from build123d import *

# Parameters (mm, degrees)
BOSS_EXTRUDE1_DEPTH      = 15
BOSS_EXTRUDE1_DEPTH_BACK = 15
SKETCH1_R                = 25
SKETCH1_R_2              = 6
SKETCH2_R                = 9.525
CUT_EXTRUDE1_START       = 15
SKETCH3_R                = 11.125
CUT_EXTRUDE1_DEPTH       = 7.2
CUT_EXTRUDE2_START       = -7.8
SKETCH4_R                = 11.125
CUT_EXTRUDE2_DEPTH       = 7.2


with BuildPart() as part:
    # Sketch1 → Boss-Extrude1 (new, two sides: drawn at the far end of the back side and taken through both)
    with BuildSketch(Plane(origin=(0, 0, 0), x_dir=(1, 0, 0), z_dir=(0, 1, 0)).offset(-BOSS_EXTRUDE1_DEPTH_BACK)):
        with Locations(Location((0, 0, 0), (0, 0, 270))):
            Circle(SKETCH1_R)
        with Locations(Location((0, 0, 0), (0, 0, 270))):
            Circle(SKETCH1_R_2, mode=Mode.SUBTRACT)
    extrude(amount=BOSS_EXTRUDE1_DEPTH + BOSS_EXTRUDE1_DEPTH_BACK)

    # Sketch2 → Cut-Revolve1 (revolve, cut)
    with BuildSketch(Plane(origin=(0, 0, 0), x_dir=(0, 0, -1), z_dir=(1, 0, 0)), mode=Mode.PRIVATE) as cut_revolve1_sk:
        with Locations((21, 0)):
            Circle(SKETCH2_R)
    revolve(cut_revolve1_sk.sketch.rotate(Axis((0, 0, 0), (0, 1, 0)), 180), axis=Axis((0, 0, 0), (0, 1, 0)), mode=Mode.SUBTRACT)

    # Sketch3 → Cut-Extrude1 (cut)
    with BuildSketch(Plane(origin=(0, 0, 0), x_dir=(1, 0, 0), z_dir=(0, 1, 0)).offset(CUT_EXTRUDE1_START)):
        with Locations(Location((0, 0, 0), (0, 0, 270))):
            Circle(SKETCH3_R)
    extrude(amount=-CUT_EXTRUDE1_DEPTH, mode=Mode.SUBTRACT)

    # Sketch4 → Cut-Extrude2 (cut)
    with BuildSketch(Plane(origin=(0, 0, 0), x_dir=(1, 0, 0), z_dir=(0, 1, 0)).offset(CUT_EXTRUDE2_START)):
        with Locations(Location((0, 0, 0), (0, 0, 270))):
            Circle(SKETCH4_R)
    extrude(amount=-CUT_EXTRUDE2_DEPTH, mode=Mode.SUBTRACT)


solid = part.part
The model under review builds one solid part; all positions refer to its coordinate system, in mm. A direction names the side the tool comes from. Coordinates: 2 decimals unless noted, no trailing zeros. Write each loop counter-clockwise with the first axis right and the second up, starting at its lowest first coordinate (ties: lowest second). Pieces come first, ordered by that corner, then holes. Notation, with made-up numbers: (83.5, -6.5) -> (122.5, -6.5) arc R30 ccw to (122.5, 25.5) -> close; hole circle Ø6 at (27.5, -4.5). An arc over 180 degrees is marked (long way). Answer in a Markdown table with one row per item.
1. We need section B-B, the plane x = 0. State the section outline as (y, z) points (3 decimals).
Answers below:
| item | result |
|---|---|
| outline | (-15, -25) -> (-8.644, -25) arc R9.525 cw (long way) to (8.644, -25) -> (15, -25) -> (15, -11.125) -> (7.8, -11.125) -> (7.8, -6) -> (-7.8, -6) -> (-7.8, -11.125) -> (-15, -11.125) -> close; (-15, 11.125) -> (-7.8, 11.125) -> (-7.8, 6) -> (7.8, 6) -> (7.8, 11.125) -> (15, 11.125) -> (15, 25) -> (8.644, 25) arc R9.525 cw (long way) to (-8.644, 25) -> (-15, 25) -> close |
2. For faces 5 (the cylindrical face through (7.509, 11.778, 23.846)), 6 (the flat face through (-5, 7.8, 5)), 7 (the flat face through (-5, -7.8, 5)), list the 3-axis set-ups (+Z, -Z, +X, -X, +Y, -Y) from which the entire face can be reached by the end or side of a thin tool; tool diameter is ignored.
Answers below:
| item | result |
|---|---|
| face 5 | +Y, -Y |
| face 6 | +Y |
| face 7 | -Y |
3. Clearance check with flat-ended pins moving along their axes: pin 1 Ø6.5 at (x, z) = (5, 1) entering from +Y; pin 2 Ø10 at (y, z) = (-0.5, 5.5) entering from -X; pin 3 Ø3 at (x, y) = (-4.5, 3) entering from +Z; pin 4 Ø9.5 at (x, z) = (0, 0) entering from +Y. State where each tip first meets the part, or that it passes through.
Answers below:
| item | result |
|---|---|
| pin 1 | stops at y = 7.8 |
| pin 2 | stops at x = -12.46 |
| pin 3 | stops at z = 11.92 |
| pin 4 | passes through |
4. We need section D-D, the plane y = -4. State the section outline as (x, z) points.
Answers below:
| item | result |
|---|---|
| outline | circle Ø24.71 at (0, 0); hole circle Ø12 at (0, 0) |
5. We need section C-C, the plane y = 10.25. State the section outline as (x, z) points (3 decimals), and give its area (3 significant figures).
Answers below:
| item | result |
|---|---|
| outline | circle Ø50 at (0, 0); hole circle Ø22.25 at (0, 0) |
| area | 1,570 mm^2 |
6. Wall thickness on probe 1 along Y at (x, z) = (-12, -17); probe 2 along X at (y, z) = (11, 0) (3 decimals); probe 3 along X at (y, z) = (1.5, 0): over which ranges is each line inside the solid? List them lowest first. Write a range as [from, to].
Answers below:
| item | result |
|---|---|
| probe 1 | y = [-15, -9.52], [9.52, 15] |
| probe 2 | x = [-25, -11.125], [11.125, 25] |
| probe 3 | x = [-11.59, -6], [6, 11.59] |
7. We need section A-A, the plane z = 0. State the section outline as (x, y) points (3 decimals).
Answers below:
| item | result |
|---|---|
| outline | (-25, -15) -> (-11.125, -15) -> (-11.125, -7.8) -> (-6, -7.8) -> (-6, 7.8) -> (-11.125, 7.8) -> (-11.125, 15) -> (-25, 15) -> (-25, 8.644) arc R9.525 cw (long way) to (-25, -8.644) -> close; (6, -7.8) -> (11.125, -7.8) -> (11.125, -15) -> (25, -15) -> (25, -8.644) arc R9.525 cw (long way) to (25, 8.644) -> (25, 15) -> (11.125, 15) -> (11.125, 7.8) -> (6, 7.8) -> close |
8. Draft analysis for pull direction X (two halves, no side actions). For faces 1 (the cylindrical face through (7.52, -11.35, -8.2)), 2 (the flat face through (-11, 15, 5)), 3 (the cylindrical face through (7.509, -11.867, 23.846)), 4 (the cylindrical face through (7.52, 11.45, -8.2)), state which applies: +X half, -X half, draft (parallel to the pull), parting line (faces both ways), or undercut.
Answers below:
| item | result |
|---|---|
| face 1 | undercut |
| face 2 | draft |
| face 3 | parting line |
| face 4 | undercut |
